from build123d import *

# Parameters (mm, degrees)
F0_R     = 20
F0_R_2   = 19
F1_DEPTH = 22
F2_R     = 20
F2_R_2   = 19
F3_DEPTH = 27
F4_R     = 20
F4_R_2   = 19
F5_DEPTH = 2


with BuildPart() as f1:
    # F0 (on Front) → F1 (new body)
    with BuildSketch(Plane.XZ):
        Circle(F0_R)
        Circle(F0_R_2, mode=Mode.SUBTRACT)
    extrude(amount=F1_DEPTH)

    # F2 (on face) → F3 (join)
    with BuildSketch(Plane.XZ.offset(22)):
        Circle(F2_R)
        Circle(F2_R_2, mode=Mode.SUBTRACT)
    extrude(amount=F3_DEPTH)

    # F4 (on face) → F5 (join)
    with BuildSketch(Plane(origin=(0, 0, 0), x_dir=(-1, 0, 0), z_dir=(0, 1, 0))):
        Circle(F4_R)
        Circle(F4_R_2, mode=Mode.SUBTRACT)
        Circle(F4_R_2)
    extrude(amount=F5_DEPTH)


solid = f1.part
Input: part model. Units: mm. Frame: model coordinates. A direction names the side the tool comes from. Coordinates: 2 decimals unless noted, no trailing zeros. Order: outer loops, then holes, each group sorted by start corner. A loop starts at its lowest first (then second) coordinate and runs counter-clockwise, first axis right, second up.
1. Cut plane A-A, the plane z = 0. Return loops of the section in (x, y).
Checked values:
outline: (-20, -49) - (-19, -49) - (-19, 0) - (19, 0) - (19, -49) - (20, -49) - (20, 2) - (-20, 2) - close
2. Cut plane C-C, the plane x = 0. Return loops of the section in (y, z).
Checked values:
outline: (-49, -20) - (2, -20) - (2, 20) - (-49, 20) - (-49, 19) - (0, 19) - (0, -19) - (-49, -19) - close
3. Ray query, line 1 along Z through (x, y) = (0, -12); line 2 along Y through (x, z) = (-9.5, 13); line 3 along Z through (x, y) = (7.5, -3). Return the intervals inside material, ascending.
Checked values:
line 1: z = -20 to -19, 19 to 20
line 2: y = 0 to 2
line 3: z = -18.54 to -17.46, 17.46 to 18.54
4. Contact query for flat-ended pins moving along their axis: P1, Ø3, axis at y = -33.5, z = 4, coming from the +X side; P2, Ø1, axis at x = 0.5, y = -3.5, coming from the +Z side; P3, Ø1, axis at x = 0, z = 3, coming from the -Y side. Output: stop coordinate, or through.
Checked values:
P1: stops at x = 19.84
P2: stops at z = 20
P3: stops at y = 0
5. Cut plane B-B, the plane y = -16.5. Return loops of the section in (x, z).
Checked values:
outline: circle Ø40 at (0, 0); hole circle Ø38 at (0, 0)
6. Access query for faces 1 (the flat face through (0, 2, 0)), 2 (the cylindrical face through (8.767, -24.157, -16.856)). Directions: +Z, -Z, +X, -X, +Y, -Y. A direction counts if a zero-diameter tool reaches every point of the face in a straight line with its end or side. Return the directions, or none.
Checked values:
face 1: +Z, -Z, +X, -X, +Y
face 2: -Y
7. Draft query along X for faces 3 (the flat face through (18, -49, -7)), 4 (the flat face through (0, 0, 0)). Return one class per face: +X half, -X half, draft (parallel to the pull), parting line (faces both ways), or undercut.
Checked values:
face 3: draft
face 4: undercut
